Here's how the part is built. I have some questions about the finished solid (model axes, mm). Face numbers are marked on the shaded views. A direction names the side the tool comes from. Give positions to 0.01 mm unless a question says otherwise; leave off trailing zeros. Write each loop counter-clockwise with the first axis right and the second up, starting at its lowest first coordinate (ties: lowest second). Pieces come first, ordered by that corner, then holes. Notation, with made-up numbers: (8.25, -16.75) - (49.25, -16.75) arc R15 cw to (49.25, 1.25) - close; hole circle Ø7 at (-17, 71). An arc over 180 degrees is marked (long way). One line per item, written item: value. Start each with the question number.
1) We'd pull the mould along Z, two halves only. Please class the marked faces 4, 5 and 6: +Z half, -Z half, draft (parallel to the pull), parting line (faces both ways), or undercut.
2) I'm going to push flat-ended pins straight in: P1, Ø2, axis at y = 4.5, z = 6, coming from the -X side; P2, Ø0.9, axis at x = -1, y = 7, coming from the +Z side; P3, Ø8, axis at x = -7, z = -7.5, coming from the +Y side (3 decimals). Where does each tip first touch, or does it pass through?
3) Imagine slicing it at B-B on x = 0. Write out the boundary of the cut face in (y, z) (3 decimals), plus the area to 3 significant figures.
4) Please list where these lines run through material, in increasing order: L1, parallel to Y at x = 5.5, z = -6 (3 decimals); L2, parallel to Y at x = -3.5, z = 1.25 (3 decimals); L3, parallel to Z at x = -8.75, y = 3.5. Write a range as [from, to].
5) Imagine slicing it at C-C on y = 1.75. Write out the boundary of the cut face in (x, z) (3 decimals), plus the area to 3 significant figures.
6) On a 3-axis mill with a long thin cutter (end or side, diameter ignored), from which of +Z, -Z, +X, -X, +Y, -Y can I reach the whole of each face in a straight line? I mean the marked faces 1, 2 and 3. Say none if no direction works.
7) Imagine slicing it at A-A on z = 0. Write out the boundary of the cut face in (x, y) (3 decimals), plus the area to 3 significant figures.
8) Imagine slicing it at D-D on x = -3.5. Write out the boundary of the cut face in (y, z) (3 decimals).
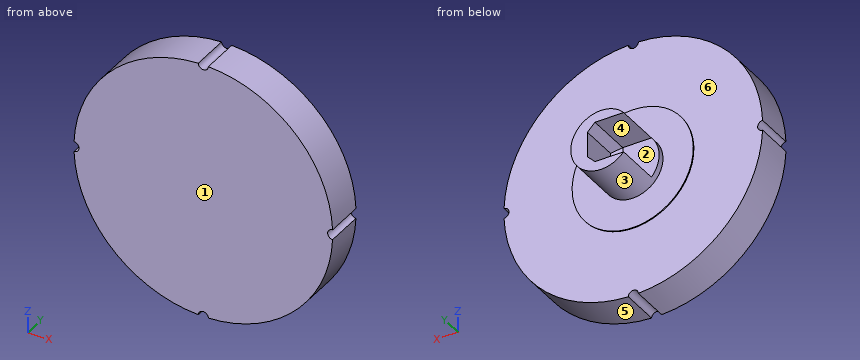
from build123d import *

# Parameters (mm, degrees)
CUT_EXTRUDE1_START      = -4.5
CUT_EXTRUDE1_DEPTH      = 4.5
CHAMFER1_SIZE           = 0.75
CUT_EXTRUDE2_DEPTH      = 21.226619836
CUT_EXTRUDE2_DEPTH_BACK = 21.226619836
SKETCH3_R               = 0.5


# Read off the part's stored shape, not the designer's step: Cut-Extrude1
with BuildPart() as part:
    # Sketch1 → Revolve1 (revolve)
    with BuildSketch(Plane.XY, mode=Mode.PRIVATE) as revolve1_sk:
        Polygon((0, 9.01), (3, 9.01), (3, 3.885), (6, 3.885), (6, 3.785), (12.805, 3.785), (12.805, 0), (0, 0), align=None)
    revolve(revolve1_sk.sketch.rotate(Axis((0, 8.620253165, 0), (0, -1, 0)), 90), axis=Axis((0, 8.620253165, 0), (0, -1, 0)))

    # Cut-Extrude1 outline → Cut-Extrude1 (cut)
    with BuildSketch(Plane(origin=(0, 9.01, 0), x_dir=(1, 0, 0), z_dir=(0, 1, 0)).offset(CUT_EXTRUDE1_START)):
        with BuildLine():
            Line((1.35, -2), (1.35, 2))
            Line((1.35, 2), (-2.236067977, 2))
            ThreePointArc((-2.236067977, 2), (-3, 0), (-2.236067977, -2))
            Line((-2.236067977, -2), (1.35, -2))
        make_face()
    extrude(amount=CUT_EXTRUDE1_DEPTH, mode=Mode.SUBTRACT)

    # Chamfer1
    chamfer1_edges = [part.edges().sort_by_distance(p)[0] for p in [
        (1.35, 6.76, 2),
        (1.35, 4.51, 0),
        (1.35, 6.76, -2),
    ]]
    chamfer(chamfer1_edges, length=CHAMFER1_SIZE)

    # Sketch3 → Cut-Extrude2 (cut, two sides: drawn at the far end of the back side and taken through both)
    with BuildSketch(Plane.XZ.offset(-CUT_EXTRUDE2_DEPTH_BACK)):
        with Locations((0, -12.805)):
            Circle(SKETCH3_R)
        with Locations((-12.805, 0)):
            Circle(SKETCH3_R)
        with Locations((12.805, 0)):
            Circle(SKETCH3_R)
        with Locations((0, 12.805)):
            Circle(SKETCH3_R)
    extrude(amount=CUT_EXTRUDE2_DEPTH + CUT_EXTRUDE2_DEPTH_BACK, mode=Mode.SUBTRACT)


solid = part.part
Numbers:
1. face 4: undercut
1. face 5: -Z half
1. face 6: draft
2. P1: x = -11.66
2. P2: z = 2.95
2. P3: y = 3.785
3. outline: (0, -12.305) - (3.785, -12.305) - (3.785, -6) - (3.885, -6) - (3.885, -3) - (9.01, -3) - (9.01, -2) - (4.51, -2) - (4.51, 2) - (9.01, 2) - (9.01, 3) - (3.885, 3) - (3.885, 6) - (3.785, 6) - (3.785, 12.305) - (0, 12.305) - close
3. area: 107 mm^2
4. L1: [0, 3.785]
4. L2: [0, 3.885]
4. L3: [-9.35, 9.35]
5. outline: (-12.795, -0.5) arc R12.805 ccw to (-0.5, -12.795) arc R0.5 cw to (0.5, -12.795) arc R12.805 ccw to (12.795, -0.5) arc R0.5 cw to (12.795, 0.5) arc R12.805 ccw to (0.5, 12.795) arc R0.5 cw to (-0.5, 12.795) arc R12.805 ccw to (-12.795, 0.5) arc R0.5 cw to start
5. area: 514 mm^2
6. face 1: +Z, -Z, +X, -X, -Y
6. face 2: -X, +Y
6. face 3: +Y
7. outline: (-12.305, 0) - (12.305, 0) - (12.305, 3.785) - (6, 3.785) - (6, 3.885) - (3, 3.885) - (3, 9.01) - (1.35, 9.01) - (1.35, 5.26) - (0.6, 4.51) - (-3, 4.51) - (-3, 3.885) - (-6, 3.885) - (-6, 3.785) - (-12.305, 3.785) - close
7. area: 106 mm^2
8. outline: (0, -12.317) - (3.785, -12.317) - (3.785, -4.873) - (3.885, -4.873) - (3.885, 4.873) - (3.785, 4.873) - (3.785, 12.317) - (0, 12.317) - close
